CAD build for the part. Positions are in the model's coordinates, mm. A direction names the side the tool comes from. Coordinates: 2 decimals unless noted, no trailing zeros. Order: outer loops, then holes, each group sorted by start corner. A loop starts at its lowest first (then second) coordinate and runs counter-clockwise, first axis right, second up. Notation, with made-up numbers: M 6.25,11 L 18.25,11 A29 cw 18.25,47 Z; hole C -6,-5 d8. An arc over 180 degrees is marked long. One line per item, written item: value.
from build123d import *

# Parameters (mm, degrees)
SKETCH1_W           = 100
SKETCH1_H           = 100
SKETCH1_R           = 7.5
BOSS_EXTRUDE1_DEPTH = 15
SKETCH2_W           = 85
SKETCH2_H           = 15
BOSS_EXTRUDE2_DEPTH = 100


with BuildPart() as part:
    # Sketch1 → Boss-Extrude1 (new body)
    with BuildSketch(Plane.XY):
        Rectangle(SKETCH1_W, SKETCH1_H)
        with Locations((0, 15)):
            Circle(SKETCH1_R, mode=Mode.SUBTRACT)
    extrude(amount=BOSS_EXTRUDE1_DEPTH)

    # Sketch2 → Boss-Extrude2 (add)
    with BuildSketch(Plane(origin=(50, 0, 0), x_dir=(0, 0, -1), z_dir=(1, 0, 0))):
        with Locations((42.5, -42.5)):
            Rectangle(SKETCH2_W, SKETCH2_H)
    extrude(amount=-BOSS_EXTRUDE2_DEPTH)


solid = part.part
Q1. Slice it at B-B (y = 15). List the corners of the cut face in (x, z).
Recorded:
outline: M -50,0 L -7.5,0 L -7.5,15 L -50,15 Z; M 7.5,0 L 50,0 L 50,15 L 7.5,15 Z
Q2. Pin check, flat tip, straight feed: pin 1 Ø5 at (x, z) = (-26, -28) entering from +Y. Stop position of the tip, or through.
Recorded:
pin 1: stops at y = -35
Q3. Slice it at D-D (y = -2). List the corners of the cut face in (x, z), plus the area to 3 significant figures.
Recorded:
outline: M -50,0 L 50,0 L 50,15 L -50,15 Z
area: 1,500 mm^2
Q4. Drill centre lines: line 1 along Y through (x, z) = (0, 11.5); line 2 along Y through (x, z) = (-22.5, -58.5); line 3 along Z through (x, y) = (5.5, 46). Where is each one in solid material? Low to high.
Recorded:
line 1: y = -50 to 7.5, 22.5 to 50
line 2: y = -50 to -35
line 3: z = 0 to 15
Q5. Slice it at A-A (x = 0). List the corners of the cut face in (y, z).
Recorded:
outline: M -50,-85 L -35,-85 L -35,0 L 7.5,0 L 7.5,15 L -50,15 Z; M 22.5,0 L 50,0 L 50,15 L 22.5,15 Z
Q6. Which spindle directions (+Z, -Z, +X, -X, +Y, -Y) get a long thin tool onto all of the face, cutting with end or side? Do faces 4 (the face through (-1, -1, 0)), 5 (the face through (1, -43, -85)). Say none if no direction does.
Recorded:
face 4: -Z, +X, -X, +Y
face 5: -Z, +X, -X, +Y, -Y
Q7. Slice it at C-C (z = -23). List the corners of the cut face in (x, y), plus the area to 3 significant figures.
Recorded:
outline: M -50,-50 L 50,-50 L 50,-35 L -50,-35 Z
area: 1,500 mm^2
Q8. Mould opens along X. For faces 1 (the face through (-1, 1, 15)), 2 (the face through (-5.5, 20.1, 7.4)), 3 (the face through (-50, -18, 2)) say: released by +X, released by -X, zero draft, split by the parting line, or undercut.
Recorded:
face 1: zero draft
face 2: undercut
face 3: released by -X
